The listing builds one solid part. Answer for the finished solid, in the listing's coordinates (mm). Face numbers are marked on the shaded views. A direction names the side the tool comes from. Round coordinates to 2 decimals unless told otherwise and drop trailing zeros. Order: outer loops, then holes, each group sorted by start corner. A loop starts at its lowest first (then second) coordinate and runs counter-clockwise, first axis right, second up. Notation, with made-up numbers: (1.25, 79.5) -> (52.25, 79.5) arc R11 ccw to (52.25, 96.5) -> close; hole circle Ø1 at (-5.75, 85.5). An arc over 180 degrees is marked (long way). Answer in a Markdown table with one row per item. Add a question column.
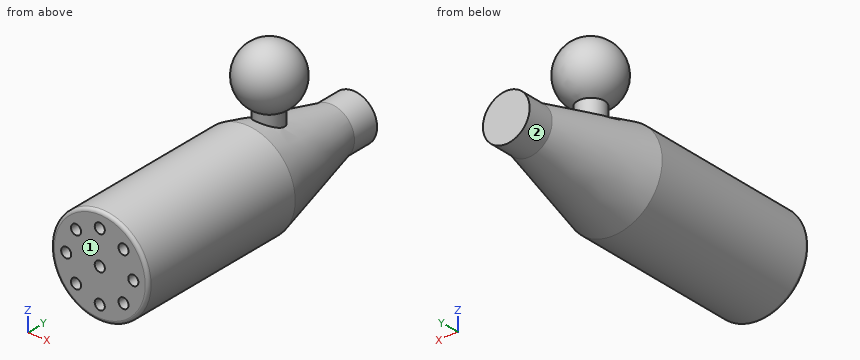
```python
from build123d import *

# Parameters (mm, degrees)
F0_R      = 5.7546875
F1_DEPTH  = 20.6375
F2_R      = 5.7546875
F3_DEPTH  = 11.90625
F3_TAPER  = 14.1
F4_R      = 2.7640442106
F5_DEPTH  = 3.175
F6_R      = 0.5953125
F7_DEPTH  = 5.08
F8_R      = 0.381
F9_R      = 1.5875
F10_DEPTH = 9.525


with BuildPart() as f1:
    # F0 (on Front) → F1 (new body)
    with BuildSketch(Plane.XZ):
        Circle(F0_R)
    extrude(amount=F1_DEPTH)

    # F2 (on face) → F3 (join)
    with BuildSketch(Plane(origin=(0, 0, 0), x_dir=(-1, 0, 0), z_dir=(0, 1, 0))):
        Circle(F2_R)
    extrude(amount=F3_DEPTH, taper=F3_TAPER)

    # F4 (on face) → F5 (join)
    with BuildSketch(Plane(origin=(0, 11.90625, 0), x_dir=(-1, 0, 0), z_dir=(0, 1, 0))):
        Circle(F4_R)
    extrude(amount=F5_DEPTH)

    # F6 (on face) → F7 (cut)
    with BuildSketch(Plane.XZ.offset(20.6375)):
        Circle(F6_R)
        with Locations((0, 3.96875)):
            Circle(F6_R)
        with Locations((-2.8063300378, 2.8063300378)):
            Circle(F6_R)
        with Locations((-3.96875, 0)):
            Circle(F6_R)
        with Locations((-2.8063300378, -2.8063300378)):
            Circle(F6_R)
        with Locations((0, -3.96875)):
            Circle(F6_R)
        with Locations((2.8063300378, -2.8063300378)):
            Circle(F6_R)
        with Locations((3.96875, 0)):
            Circle(F6_R)
        with Locations((2.8063300378, 2.8063300378)):
            Circle(F6_R)
    extrude(amount=-F7_DEPTH, mode=Mode.SUBTRACT)

    # F8
    f8_edges = [f1.edges().sort_by_distance(p)[0] for p in [
        (-5.754687, -20.6375, 0),
    ]]
    fillet(f8_edges, radius=F8_R)

    # F9 (on Top) → F10 (join)
    with BuildSketch(Plane.XY):
        with Locations((0, 3.175)):
            Circle(F9_R)
    extrude(amount=F10_DEPTH)

    # F11 (on Right) → F12 (revolve)
    with BuildSketch(Plane.YZ):
        with BuildLine():
            Line((3.2164233271, 13.096875), (3.2164233271, 5.953125))
            ThreePointArc((3.2164233271, 5.953125), (6.7882983271, 9.525), (3.2164233271, 13.096875))
        make_face()
    revolve(axis=Axis((0, 3.2164233271, 9.525), (0, 0, 1)))


solid = f1.part
```
1. For the marked faces 1 and 2, determine the directions among +Z, -Z, +X, -X, +Y, -Y from which every point of the face is accessible in a straight line to the end or side of a thin tool.
2. Each of these flat-tipped pins is pushed along its axis until it touches: pin 1 (3 mm diameter, centred on x = -4.5, y = -5, fed in from -Z); pin 2 (0.6 mm diameter, centred on x = 0, z = 4, fed in from -Y); pin 3 (3 mm diameter, centred on x = -2.5, y = -0.5, fed in from -Z). Where does it stop, or does it pass through?
3. The part is cut by section B-B (y = -7.5). Give the vertices of the cut face in (x, z).
4. Straight lines are drawn through the part: line 1 along X through (y, z) = (0.5, 4.5); line 2 along Z through (x, y) = (-3.5, -16); line 3 along Z through (x, y) = (2.5, 1.5). For each, find the intervals that lie inside material, in ascending order.
5. The part is cut by section A-A (x = 0). Give the vertices of the cut face in (y, z) (1 decimal), then the cut area to 3 significant figures.
Report:
| question | item | result |
|---|---|---|
| 1 | face 1 | +Z, -Z, +X, -X, -Y |
| 1 | face 2 | +Y |
| 2 | pin 1 | stops at z = -4.91 |
| 2 | pin 2 | stops at y = -15.56 |
| 2 | pin 3 | stops at z = -5.67 |
| 3 | outline | circle Ø11.51 at (0, 0) |
| 4 | line 1 | x = -3.38 to 3.38 |
| 4 | line 2 | z = -4.57 to -0.37, 0.37 to 4.57 |
| 4 | line 3 | z = -4.76 to 4.76, 7.64 to 11.41 |
| 5 | outline | (-20.6, -5.4) arc R0.4 ccw to (-20.3, -5.8) -> (0, -5.8) -> (11.9, -2.8) -> (15.1, -2.8) -> (15.1, 2.8) -> (11.9, 2.8) -> (4.8, 4.6) -> (4.8, 6.3) arc R3.6 ccw (long way) to (1.6, 6.3) -> (1.6, 5.4) -> (0, 5.8) -> (-20.3, 5.8) arc R0.4 ccw to (-20.6, 5.4) -> (-20.6, 4.6) -> (-15.6, 4.6) -> (-15.6, 3.4) -> (-20.6, 3.4) -> (-20.6, 0.6) -> (-15.6, 0.6) -> (-15.6, -0.6) -> (-20.6, -0.6) -> (-20.6, -3.4) -> (-15.6, -3.4) -> (-15.6, -4.6) -> (-20.6, -4.6) -> close |
| 5 | area | 382 mm^2 |
